Could you check a few things on this model? Use its own coordinates, in mm. A direction names the side the tool comes from. Coordinates: 2 decimals unless noted, no trailing zeros. Write each loop counter-clockwise with the first axis right and the second up, starting at its lowest first coordinate (ties: lowest second). Pieces come first, ordered by that corner, then holes.
Item 1: I want a section at A-A on y = 21.25. Please give me the cut outline in (x, z), then the cut area to 4 significant figures.
Item 2: If I drill on probe 1 along X at (y, z) = (-1, 80.5); probe 2 along Z at (x, y) = (37, -30); probe 3 along Y at (x, z) = (-29.5, 77), over which ranges is the centre line in solid material (lowest first)?
Item 3: I want a section at D-D on y = 6. Please give me the cut outline in (x, z), then the cut area to 4 significant figures.
Item 4: I want a section at B-B on z = 8. Please give me the cut outline in (x, y).
Item 5: For P1, Ø9.5, axis at x = 37, z = 8, coming from the +Y side; P2, Ø5, axis at x = -37, y = 21.25, coming from the -Z side; P3, Ø1, axis at x = -8, y = -18, coming from the -Z side, each with a flat end and sliding along its axis, tell me the tip position at first contact or that it passes through.
Item 6: Thinking about a two-plate mould opening in X: for faces 3 (the flat face through (-45, 0, 44)), 4 (the cylindrical face through (-39.997, 21.382, 89.26)), 5 (the flat face through (-1, -30.75, 44)), which applies, +X half, -X half, draft (parallel to the pull), parting line (faces both ways), or undercut?
Item 7: Which directions (+Z, -Z, +X, -X, +Y, -Y) give clear straight access to the entire face, cutting with the end or side of a thin tool? Please do faces 1 (the flat face through (-44, 29.25, 45)), 2 (the flat face through (-1, 0, 88.5)).
Item 8: I want a section at C-C on x = 37. Please give me the cut outline in (y, z), then the cut area to 3 significant figures.
Autodesk Inventor part; units mm, degrees
ref_plane "Work Plane2" through (-45.2602, 13.6363, 90) normal (0, 0, 1) x (1, 0, 0)
ref_plane "Work Plane3" through (-81.5561, 29.25, -36.5561) normal (0, -1, 0) x (1, 0, 0)
ref_plane "Work Plane4" through (-81.5561, 29.25, -36.5561) normal (0, -1, 0) x (1, 0, 0)
ref_plane "Work Plane1" through (0.1672, 0, 0) normal (0, 0, 1) x (1, 0, 0)
sketch "Sketch1" plane through (0.1672, 0, 0) normal (0, 0, 1) x (1, 0, 0)
  line L0 (-45.1672, 29.25) -> (44.8328, 29.25)
  line L1 (-45.1672, 29.25) -> (-45.1672, -30.75)
  line L2 (-45.1672, -30.75) -> (44.8328, -30.75)
  line L3 (44.8328, -30.75) -> (44.8328, 29.25)
  circle A0 centre (-37.1672, -22.75) radius 3
  line L4 (44.8328, -30.75) -> (-45.1672, -30.75)
  line L5 (-45.1672, -30.75) -> (-45.1672, -29.25)
  line L6 (-45.1672, -29.25) -> (44.8328, -29.25)
  line L7 (44.8328, -29.25) -> (44.8328, -30.75)
  point P0 (-0.1672, 0)
  dimension "d0" = 1.5
ref_plane "Work Plane2" through (-45.2602, 13.6363, 90) normal (0, 0, 1) x (1, 0, 0)
extrude "Extrusion1" add sketch "Sketch1" along normal up to surface (90 mm away) contours L6 L3 L2 L1
sketch "Sketch2" plane through (-45, -29.25, 0) normal (0, 1, 0) x (1, 0, 0)
  line L0 (90, 0) -> (90, -90)
  line L1 (0, 0) -> (0, -90)
  line L2 (90, -90) -> (0, -90)
  line L3 (0, -90) -> (0, -88.5)
  line L4 (0, -88.5) -> (90, -88.5)
  line L5 (90, -88.5) -> (90, -90)
  point P0 (45, 0)
  dimension "d3" = 1.5
ref_plane "Work Plane3" through (-81.5561, 29.25, -36.5561) normal (0, -1, 0) x (1, 0, 0)
extrude "Extrusion2" add sketch "Sketch2" along normal up to surface (58.5 mm away)
sketch "Sketch4" plane through (-45, -29.25, 0) normal (0, 1, 0) x (1, 0, 0)
  line L0 (90, 0) -> (90, -88.5)
  line L1 (90, 0) -> (0, 0)
  line L2 (90, -88.5) -> (88.5, -88.5)
  line L3 (88.5, -88.5) -> (88.5, 0)
  line L4 (88.5, 0) -> (90, 0)
  line L5 (90, 0) -> (90, -88.5)
  line L6 (0, 0) -> (0, -88.5)
  line L7 (0, -88.5) -> (1.5, -88.5)
  line L8 (1.5, -88.5) -> (1.5, 0)
  line L9 (1.5, 0) -> (0, 0)
  line L10 (0, 0) -> (0, -88.5)
  point P0 (45, 0)
  dimension "d7" = 1.5
  dimension "d8" = 1.5
ref_plane "Work Plane4" through (-81.5561, 29.25, -36.5561) normal (0, -1, 0) x (1, 0, 0)
extrude "Extrusion3" add sketch "Sketch4" along normal up to surface (58.5 mm away)
sketch "Sketch5" plane through (-45, -30.75, 0) normal (0, -1, 0) x (1, 0, 0)
  circle A0 centre (82, 8) radius 3
  point P0 (45, 0)
extrude "Extrusion4" cut sketch "Sketch5" against normal up to next
sketch "Sketch6" plane through (-45, -30.75, 90) normal (0, 0, 1) x (1, 0, 0)
  circle A0 centre (8, 52) radius 3
  point P0 (45, 30.75)
extrude "Extrusion5" cut sketch "Sketch6" against normal up to next
properties part number "fixação chave geral"
Response values:
1. outline: (-45, 0) - (-43.5, 0) - (-43.5, 88.5) - (-40, 88.5) - (-40, 90) - (-45, 90) - close; (-34, 88.5) - (43.5, 88.5) - (43.5, 0) - (45, 0) - (45, 90) - (-34, 90) - close
1. area: 391.5 mm2
2. probe 1: x = -45 to -43.5, 43.5 to 45
2. probe 2: z = 0 to 5, 11 to 90
2. probe 3: y = -30.75 to -29.25
3. outline: (-45, 0) - (-43.5, 0) - (-43.5, 88.5) - (43.5, 88.5) - (43.5, 0) - (45, 0) - (45, 90) - (-45, 90) - close
3. area: 400.5 mm2
4. outline: (-45, -30.75) - (34, -30.75) - (34, -29.25) - (-43.5, -29.25) - (-43.5, 29.25) - (-45, 29.25) - close; (40, -30.75) - (45, -30.75) - (45, 29.25) - (43.5, 29.25) - (43.5, -29.25) - (40, -29.25) - close
5. P1: stops at y = -29.25
5. P2: passes through
5. P3: stops at z = 88.5
6. face 3: -X half
6. face 4: undercut
6. face 5: draft
7. face 1: +Z, -Z, +X, -X, +Y
7. face 2: -Z, +Y
8. outline: (-30.75, 0) - (-29.25, 0) - (-29.25, 5) - (-30.75, 5) - close; (-30.75, 11) - (-29.25, 11) - (-29.25, 88.5) - (29.25, 88.5) - (29.25, 90) - (-30.75, 90) - close
8. area: 214 mm2
